Geometry check sheet. Reference: drawing and pictorial views, mm from the part's lowest x, y, z. A direction names the side the tool comes from. Round coordinates to 2 decimals unless told otherwise and drop trailing zeros. Order: outer loops, then holes, each group sorted by start corner. A loop starts at its lowest first (then second) coordinate and runs counter-clockwise, first axis right, second up. Notation, with made-up numbers: (79, 32) -> (84, 32) arc R17 ccw to (84, 61) -> close; hole circle Ø11 at (-24, -9). An arc over 180 degrees is marked (long way). Put each result on its own line as item: value.
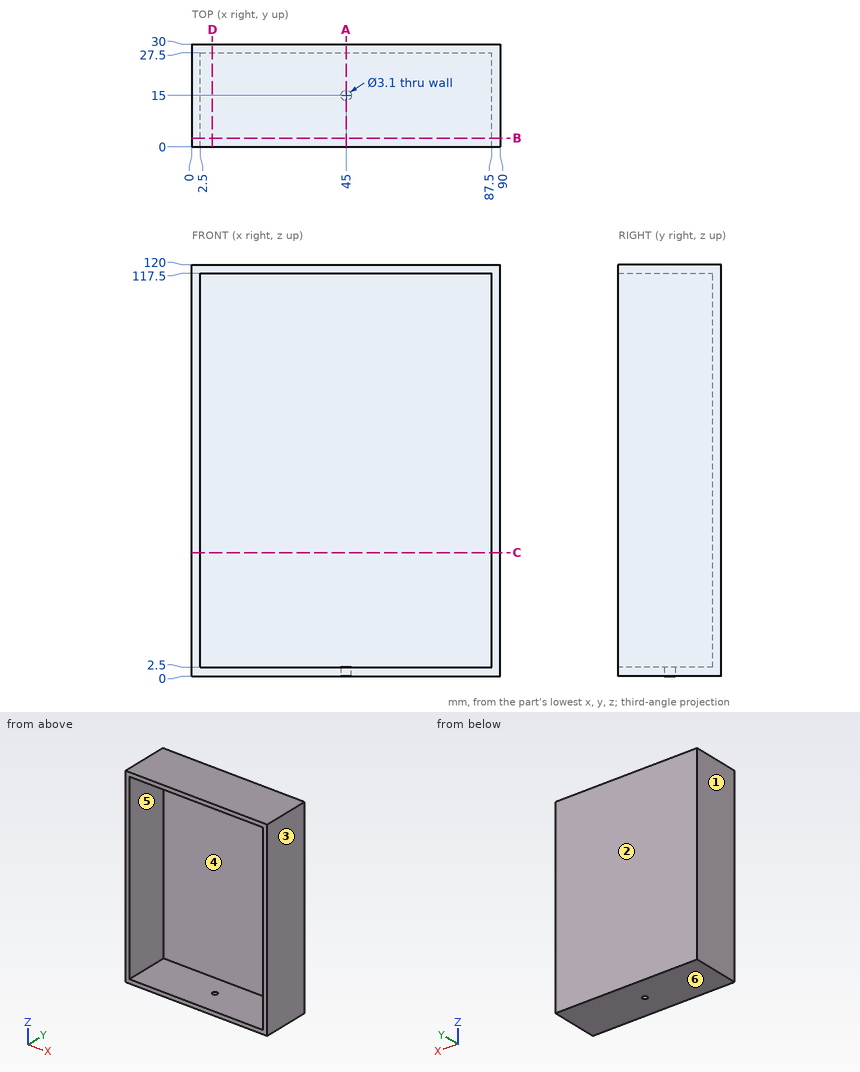
Item 1: Release check for a two-part mould opening along X. For the marked faces 1, 2, 3 and 4 record: pulls with the +X half, pulls with the -X half, needs draft (parallel to the pull), parting line crosses it, or undercut.
Geometry check:
face 1: pulls with the -X half
face 2: needs draft
face 3: pulls with the +X half
face 4: undercut
Item 2: Sectioned sample at C-C, the plane z = 36. Record the boundary of the cut face in (x, y).
Geometry check:
outline: (0, 0) -> (2.5, 0) -> (2.5, 27.5) -> (87.5, 27.5) -> (87.5, 0) -> (90, 0) -> (90, 30) -> (0, 30) -> close
Item 3: Material ranges on line 1 along X through (y, z) = (18.5, 69.5); line 2 along Z through (x, y) = (55, 12.75); line 3 along Y through (x, z) = (45, 1), recorded low to high.
Geometry check:
line 1: 0 to 2.5, 87.5 to 90
line 2: 0 to 2.5, 117.5 to 120
line 3: 0 to 13.45, 16.55 to 30
Item 4: Tool access check on the marked faces 5 and 6. Record the directions out of +Z, -Z, +X, -X, +Y, -Y that give a thin tool (end or side, any length) a straight path to the whole face; none if there is none.
Geometry check:
face 5: -Y
face 6: -Z, +X, -X, +Y, -Y
Item 5: Sectioned sample at B-B, the plane y = 2.5. Record the boundary of the cut face in (x, z), then the cut area to 4 significant figures.
Geometry check:
outline: (0, 0) -> (90, 0) -> (90, 120) -> (0, 120) -> close; hole (2.5, 2.5) -> (87.5, 2.5) -> (87.5, 117.5) -> (2.5, 117.5) -> close
area: 1,025 mm2
Item 6: Sectioned sample at A-A, the plane x = 45. Record the boundary of the cut face in (y, z), then the cut area to 3 significant figures.
Geometry check:
outline: (0, 0) -> (13.45, 0) -> (13.45, 2.5) -> (0, 2.5) -> close; (0, 117.5) -> (27.5, 117.5) -> (27.5, 2.5) -> (16.55, 2.5) -> (16.55, 0) -> (30, 0) -> (30, 120) -> (0, 120) -> close
area: 430 mm2
Item 7: Sectioned sample at D-D, the plane x = 6. Record the boundary of the cut face in (y, z).
Geometry check:
outline: (0, 0) -> (30, 0) -> (30, 120) -> (0, 120) -> (0, 117.5) -> (27.5, 117.5) -> (27.5, 2.5) -> (0, 2.5) -> close
Item 8: Depth check by flat-ended pin: pin 1 Ø2 at (x, z) = (74.5, 71) entering from -Y. Enter the tip coordinate at first touch or a pass-through.
Geometry check:
pin 1: y = 27.5
